Autodesk Fusion 360 part; units mm, degrees
sketch "Skizze1" plane through (0, 0, 0) normal (0, 1, 0) x (1, 0, 0)
  line L0 (43, 27) -> (-43, 27)
  line L1 (-43, 27) -> (-43, -27)
  line L2 (-43, -27) -> (43, -27)
  line L3 (43, -27) -> (43, 27)
  line L4 (43, 27) -> (-43, -27) construction
  line L5 (-43, 27) -> (43, -27) construction
  dimension "d1" = 54
  dimension "d2" = 86
extrude "Extrusion1" add sketch "Skizze1" along normal blind 2
fillet "Abrundung1" radius 3 4 edges at (43, 1, -27) (43, 1, 27) (-43, 1, 27) (-43, 1, -27)
sketch "Skizze2" plane through (0, 2, 0) normal (0, 1, 0) x (-1, 0, 0)
  arc A0 (40, -27) -> (43, -24) centre (40, -24) ccw
  line L0 (43, -24) -> (43, 24)
  arc A1 (43, 24) -> (40, 27) centre (40, 24) ccw
  line L1 (40, 27) -> (-40, 27)
  arc A2 (-40, 27) -> (-43, 24) centre (-40, 24) ccw
  line L2 (-43, 24) -> (-43, -24)
  arc A3 (-43, -24) -> (-40, -27) centre (-40, -24) ccw
  line L3 (-40, -27) -> (40, -27)
  line L4 (37.5, -6) -> (-37.5, -6)
  line L5 (-37.5, -6) -> (-37.5, 6)
  line L6 (-37.5, 6) -> (37.5, 6)
  line L7 (37.5, 6) -> (37.5, -6)
  line L8 (37.5, -6) -> (-37.5, 6) construction
  line L9 (-37.5, -6) -> (37.5, 6) construction
  dimension "d7" = 12
  dimension "d8" = 75
extrude "Extrusion2" cut sketch "Skizze2" against normal blind 1.2 contours L4 L5 L6 L7
fillet "Abrundung2" radius 1 4 edges at (37.5, 1.4, -6) (37.5, 1.4, 6) (-37.5, 1.4, -6) (-37.5, 1.4, 6)
Can you work these out from the model? Positions are in its coordinate system, mm. Coordinates: 2 decimals unless noted, no trailing zeros. Loops run counter-clockwise (first coordinate to the right, second up) from the corner with the lowest first, then second, coordinate; pieces in that order, holes last. Notation, with made-up numbers: (75, 38) - (131, 38) arc R16 ccw to (131, 48) - close; hole circle Ø8 at (46.25, 70.5). An arc over 180 degrees is marked (long way). Use a Markdown table: item, result.
Item 1: If I drill on probe 1 along Z at (x, y) = (-35, 1.65); probe 2 along X at (y, z) = (1.75, -5); probe 3 along Y at (x, z) = (6, -5), over which ranges is the centre line in solid material (lowest first)? Write a range as from..to.
Numbers:
| item | result |
|---|---|
| probe 1 | z = -27..-6, 6..27 |
| probe 2 | x = -43..-37.5, 37.5..43 |
| probe 3 | y = 0..0.8 |
Item 2: We'd pull the mould along X, two halves only. Please class faces 1 (the face through (42.14, 1.01, -26.1)), 2 (the face through (1, 1, -27)), 3 (the face through (1, 0.8, 0)): released by +X, released by -X, zero draft, split by the parting line, or undercut.
Numbers:
| item | result |
|---|---|
| face 1 | released by +X |
| face 2 | zero draft |
| face 3 | undercut |
Item 3: Will this pin go through, and if not, where does the flat tip stop? pin 1 (10 mm diameter, centred on x = -21, z = 3.5, fed in from -Y).
Numbers:
| item | result |
|---|---|
| pin 1 | stops at y = 0 |
Item 4: I want a section at C-C on x = 22.5. Please give me the cut outline in (y, z), and give its area (3 significant figures).
Numbers:
| item | result |
|---|---|
| outline | (0, -27) - (2, -27) - (2, -6) - (0.8, -6) - (0.8, 6) - (2, 6) - (2, 27) - (0, 27) - close |
| area | 93.6 mm2 |
Item 5: I want a section at A-A on y = 1.7. Please give me the cut outline in (x, z).
Numbers:
| item | result |
|---|---|
| outline | (-43, -24) arc R3 ccw to (-40, -27) - (40, -27) arc R3 ccw to (43, -24) - (43, 24) arc R3 ccw to (40, 27) - (-40, 27) arc R3 ccw to (-43, 24) - close; hole (-37.5, -5) arc R1 ccw to (-36.5, -6) - (36.5, -6) arc R1 ccw to (37.5, -5) - (37.5, 5) arc R1 ccw to (36.5, 6) - (-36.5, 6) arc R1 ccw to (-37.5, 5) - close |
Item 6: I want a section at B-B on z = -1. Please give me the cut outline in (x, y).
Numbers:
| item | result |
|---|---|
| outline | (-43, 0) - (43, 0) - (43, 2) - (37.5, 2) - (37.5, 0.8) - (-37.5, 0.8) - (-37.5, 2) - (-43, 2) - close |
